```python
from build123d import *

# Parameters (mm, degrees)
FILLET1_R               = 0.5
FILLET2_R               = 0.2
SKETCH2_R               = 1.2
CUT_EXTRUDE1_DEPTH      = 6.25
CUT_EXTRUDE1_DEPTH_BACK = 6.25
BOSS_EXTRUDE1_DEPTH     = 3


with BuildPart() as part:
    # Sketch1 → Revolve1 (revolve)
    with BuildSketch(Plane.XY):
        Polygon((11, 2.15), (11, 3.5), (-8, 3.5), (-8, 5.25), (-11, 5.25), (-11, 3.5), (-9.524, 3.5), (-9.524, 2.15), align=None)
    revolve(axis=Axis((-11, 0, 0), (1, 0, 0)))

    # Fillet1
    fillet1_edges = [part.edges().sort_by_distance(p)[0] for p in [
        (-8, -3.5, 0),
    ]]
    fillet(fillet1_edges, radius=FILLET1_R)

    # Fillet2
    fillet2_edges = [part.edges().sort_by_distance(p)[0] for p in [
        (-9.524, -3.5, 0),
    ]]
    fillet(fillet2_edges, radius=FILLET2_R)

    # Sketch2 → Cut-Extrude1 (cut, two sides)
    with BuildSketch(Plane(origin=(0, 0, 0), x_dir=(1, 0, 0), z_dir=(0, 1, 0))) as cut_extrude1_sk:
        with Locations((1.75, 0)):
            Circle(SKETCH2_R)
    extrude(amount=CUT_EXTRUDE1_DEPTH, mode=Mode.SUBTRACT)
    extrude(cut_extrude1_sk.sketch, amount=-CUT_EXTRUDE1_DEPTH_BACK, mode=Mode.SUBTRACT)

    # Sketch3 → Boss-Extrude1 (add)
    with BuildSketch(Plane.ZY.offset(11)):
        with BuildLine():
            ThreePointArc((1.011232478, 5.151689905), (0, 6.266), (-1.011232478, 5.151689905))
            ThreePointArc((-1.011232478, 5.151689905), (0, 5.25), (1.011232478, 5.151689905))
        make_face()
        with BuildLine():
            ThreePointArc((4.967110569, 1.700091937), (5.42651518, 3.133), (3.955878091, 3.451597968))
            ThreePointArc((3.955878091, 3.451597968), (4.54663337, 2.625), (4.967110569, 1.700091937))
        make_face()
        with BuildLine():
            ThreePointArc((3.955878091, -3.451597968), (5.42651518, -3.133), (4.967110569, -1.700091937))
            ThreePointArc((4.967110569, -1.700091937), (4.54663337, -2.625), (3.955878091, -3.451597968))
        make_face()
        with BuildLine():
            ThreePointArc((-1.011232478, -5.151689905), (0, -6.266), (1.011232478, -5.151689905))
            ThreePointArc((1.011232478, -5.151689905), (0, -5.25), (-1.011232478, -5.151689905))
        make_face()
        with BuildLine():
            ThreePointArc((-4.967110569, -1.700091937), (-5.42651518, -3.133), (-3.955878091, -3.451597968))
            ThreePointArc((-3.955878091, -3.451597968), (-4.54663337, -2.625), (-4.967110569, -1.700091937))
        make_face()
        with BuildLine():
            ThreePointArc((-3.955878091, 3.451597968), (-5.42651518, 3.133), (-4.967110569, 1.700091937))
            ThreePointArc((-4.967110569, 1.700091937), (-4.54663337, 2.625), (-3.955878091, 3.451597968))
        make_face()
    extrude(amount=-BOSS_EXTRUDE1_DEPTH)


solid = part.part
```
Work out the finished part from the listing and answer in its coordinate system (mm). A direction names the side the tool comes from. Coordinates: 2 decimals unless noted, no trailing zeros. Write each loop counter-clockwise with the first axis right and the second up, starting at its lowest first coordinate (ties: lowest second). Pieces come first, ordered by that corner, then holes.
Q1. A cutting plane is placed at D-D, the plane x = 8.5. Give the vertices of the cut face in (y, z), then the cut area to 3 significant figures.
Q2. Determine the mould class of faces 1 (the face through (-8, 3, -3)), 2 (the face through (-9.52, 4.53, -2.65)), 3 (the face through (-9.521, -3.153, 5.414)), 4 (the face through (0.882, -1.706, -1.308)) for opening direction Y: released by +Y, released by -Y, zero draft, split by the parting line, or undercut.
Q3. A cutting plane is placed at C-C, the plane z = 0.5. State how many separate pieces and enclosed holes the cut face has, then the cut area to 3 significant figures.
Q4. Each of these flat-tipped pins is pushed along its axis until it touches: pin 1 Ø1.5 at (x, y) = (-0.5, 0) entering from -Z; pin 2 Ø3.5 at (y, z) = (0.5, -0.5) entering from -X; pin 3 Ø3.5 at (y, z) = (0, 0) entering from +X; pin 4 Ø3 at (x, z) = (1.75, 0) entering from +Y. Where does it stop, or does it pass through?
Q5. A cutting plane is placed at A-A, the plane y = 0. Give the vertices of the cut face in (x, z), then the cut area to 3 significant figures.
Q6. Which of the six approach directions +Z, -Z, +X, -X, +Y, -Y give full straight-line access (tool end or side, diameter ignored) to faces 5 (the face through (1.62, 1.615, -3.105)), 6 (the face through (0.55, -2.63, -0.05)), 7 (the face through (-10.353, 3.233, -1.341))?
Q7. Find the intervals of material crossed by line 1 (Y direction, x = 5.25, z = 0); line 2 (X direction, y = 1.75, z = 1.75), in increasing order.
Q8. A cutting plane is placed at B-B, the plane x = 1.75. Give the vertices of the cut face in (y, z).
Findings below:
1. outline: circle Ø7 at (0, 0); hole circle Ø4.3 at (0, 0)
1. area: 24.0 mm2
2. face 1: zero draft
2. face 2: released by +Y
2. face 3: undercut
2. face 4: undercut
3. separate pieces: 4
3. enclosed holes: 0
3. area: 66.5 mm2
4. pin 1: stops at z = -3.5
4. pin 2: stops at x = -9.52
4. pin 3: passes through
4. pin 4: stops at y = 3.5
5. outline: (-11, -5.25) - (-8, -5.25) - (-8, -4) arc R0.5 cw to (-7.5, -3.5) - (11, -3.5) - (11, -2.15) - (-9.52, -2.15) - (-9.52, -3.3) arc R0.2 cw to (-9.72, -3.5) - (-11, -3.5) - close; (-11, 3.5) - (-9.72, 3.5) arc R0.2 cw to (-9.52, 3.3) - (-9.52, 2.15) - (11, 2.15) - (11, 3.5) - (-7.5, 3.5) arc R0.5 cw to (-8, 4) - (-8, 5.25) - (-11, 5.25) - close
5. area: 66.0 mm2
6. face 5: +X
6. face 6: +Y, -Y
6. face 7: -X
7. line 1: y = -3.5 to -2.15, 2.15 to 3.5
7. line 2: x = -9.52 to 11
8. outline: (-3.29, -1.2) arc R3.5 ccw to (3.29, -1.2) - (1.78, -1.2) arc R2.15 cw to (-1.78, -1.2) - close; (-3.29, 1.2) - (-1.78, 1.2) arc R2.15 cw to (1.78, 1.2) - (3.29, 1.2) arc R3.5 ccw to start
